Part model, mm, in its own coordinate system. Face numbers are marked on the shaded views. Round coordinates to 2 decimals unless told otherwise and drop trailing zeros. Loops run counter-clockwise (first coordinate to the right, second up) from the corner with the lowest first, then second, coordinate; pieces in that order, holes last. Notation, with made-up numbers: (-18.5, 5) - (-14.5, 5) arc R36 ccw to (-14.5, 43) - close; hole circle Ø4 at (34.5, 84). An arc over 180 degrees is marked (long way). Write each question's results on one line, items separated by ' | '. Start each with the question number.
(1) Cut at B-B, the plane z = -59.5. List the corners of the cut face in (x, y).
(2) Mould opens along X. For the marked faces 1 and 2 say: released by +X, released by -X, zero draft, split by the parting line, or undercut.
(3) Cut at C-C, the plane x = 11.5. List the corners of the cut face in (y, z).
(4) Flat gauge pin, fed straight in: P1, Ø13.5, axis at x = 8.5, z = -42.5, coming from the +Y side. Where does the tip first touch, or does it go through?
(5) Drill centre lines: L1, parallel to Y at x = 32.5, z = 1; L2, parallel to X at y = 21.5, z = -153; L3, parallel to X at y = 29.95, z = -38.1. Where is each one in solid material? Low to high.
(6) Cut at A-A, the plane y = 20. List the corners of the cut face in (x, z), then the cut area to 3 significant figures.
(7) Cut at D-D, the plane z = -23. List the corners of the cut face in (x, y).
Autodesk Inventor part; units mm, degrees
ref_plane "YZ Plane" through (0, 0, 0) normal (1, 0, 0) x (0, 1, 0)
ref_plane "XZ Plane" through (0, 0, 0) normal (0, 1, 0) x (-1, 0, 0)
ref_plane "XY Plane" through (0, 0, 0) normal (0, 0, 1) x (1, 0, 0)
sketch "Sketch1" plane through (0, 0, 0) normal (0, 0, 1) x (1, 0, 0)
  line L0 (37.2518, 31.5045) -> (-13.5482, 31.5045)
  line L1 (-13.5482, 31.5045) -> (-13.5482, 6.1045)
  line L2 (-13.5482, 6.1045) -> (37.2518, 6.1045)
  line L3 (37.2518, 6.1045) -> (37.2518, 31.5045)
  line L4 (34.0768, 28.3295) -> (-10.3732, 28.3295)
  line L5 (-10.3732, 28.3295) -> (-10.3732, 9.2795)
  line L6 (-10.3732, 9.2795) -> (34.0768, 9.2795)
  line L7 (34.0768, 9.2795) -> (34.0768, 28.3295)
  point P0 (0, 0)
  dimension "d0" = 50.8
  dimension "d1" = 25.4
  dimension "d2" = 3.175
extrude "Extrusion1" add sketch "Sketch1" against normal blind 177.8 and the other way blind 88.9
sketch "Sketch2" plane through (-13.5482, 31.5045, -177.8) normal (0, 1, 0) x (1, 0, 0)
  circle A0 centre (25.4, -139.7) radius 19.05
  line L0 (50.8, -266.7) -> (0, -266.7)
  point P0 (13.5482, -177.8)
  point P1 (25.4, -266.7)
  dimension "d7" = 38.1
  dimension "d8" = 127
extrude "Extrusion2" cut sketch "Sketch2" against normal blind 3.175
properties part number "Motor Mount"
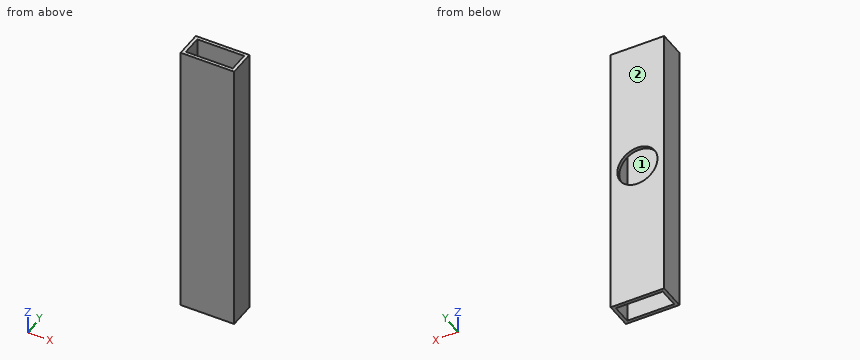
A:
1) outline: (-13.55, 6.1) - (37.25, 6.1) - (37.25, 31.5) - (-13.55, 31.5) - close; hole (-10.37, 9.28) - (34.08, 9.28) - (34.08, 28.33) - (-10.37, 28.33) - close
2) face 1: undercut | face 2: zero draft
3) outline: (6.1, -177.8) - (9.28, -177.8) - (9.28, 88.9) - (6.1, 88.9) - close; (28.33, -177.8) - (31.5, -177.8) - (31.5, -57.15) - (28.33, -57.15) - close; (28.33, -19.05) - (31.5, -19.05) - (31.5, 88.9) - (28.33, 88.9) - close
4) P1: y = 9.28
5) L1: 6.1 to 9.28, 28.33 to 31.5 | L2: -13.55 to -10.37, 34.08 to 37.25 | L3: -13.55 to -7.2, 30.9 to 37.25
6) outline: (-13.55, -177.8) - (-10.37, -177.8) - (-10.37, 88.9) - (-13.55, 88.9) - close; (34.08, -177.8) - (37.25, -177.8) - (37.25, 88.9) - (34.08, 88.9) - close | area: 1,690 mm2
7) outline: (-13.55, 6.1) - (37.25, 6.1) - (37.25, 31.5) - (23.47, 31.5) - (23.47, 28.33) - (34.08, 28.33) - (34.08, 9.28) - (-10.37, 9.28) - (-10.37, 28.33) - (0.24, 28.33) - (0.24, 31.5) - (-13.55, 31.5) - close
